from build123d import *

# Parameters (mm, degrees)
SKETCH_R        = 90
PAD_DEPTH       = 1.6
SKETCH001_R     = 90
SKETCH001_R_2   = 88
PAD001_DEPTH    = 20
SKETCH006_R     = 5.2
POCKET_DEPTH    = 6
PAD006_DEPTH    = 20
POCKET001_DEPTH = 8
SKETCH008_R     = 5.2
PAD007_DEPTH    = 1.8
SKETCH057_R     = 1.396673
SKETCH057_R_2   = 1.389292
SKETCH057_W     = 5
SKETCH057_H     = 5
PAD037_DEPTH    = 20


with BuildPart() as part:
    # Sketch → Pad (new body)
    with BuildSketch(Plane.XY):
        Circle(SKETCH_R)
    extrude(amount=PAD_DEPTH)

    # Sketch001 (on Face3 of Pad) → Pad001 (join)
    with BuildSketch(Plane.XY.offset(1.6)):
        Circle(SKETCH001_R)
        Circle(SKETCH001_R_2, mode=Mode.SUBTRACT)
    extrude(amount=PAD001_DEPTH)

    # Sketch006 (on Face2 of ShapeBinder) → Pocket (cut)
    with BuildSketch(Plane(origin=(0, 90, 8), x_dir=(1, 0, 0), z_dir=(0, 1, 0))):
        Circle(SKETCH006_R)
    extrude(amount=-POCKET_DEPTH, mode=Mode.SUBTRACT)

    # Sketch007 (on Face7 of Pocket) → Pad006 (join)
    with BuildSketch(Plane.XY.offset(1.6)):
        with BuildLine():
            ThreePointArc((7, 87.721149), (0, 88), (-7, 87.721149))
            Line((-7, 87.721149), (-7, 84))
            Line((-7, 84), (7, 84))
            Line((7, 84), (7, 87.721149))
        make_face()
    extrude(amount=PAD006_DEPTH)

    # Sketch006 (on Face2 of ShapeBinder) → Pocket001 (cut)
    with BuildSketch(Plane(origin=(0, 90, 8), x_dir=(1, 0, 0), z_dir=(0, 1, 0))):
        Circle(SKETCH006_R)
    extrude(amount=-POCKET001_DEPTH, mode=Mode.SUBTRACT)

    # Sketch008 (on Face13 of Pocket001) → Pad007 (join)
    with BuildSketch(Plane.XZ.offset(-84)):
        with Locations((0, 8)):
            Circle(SKETCH008_R)
        with BuildLine():
            ThreePointArc((1.843231, 4.45), (4, 8), (1.843231, 11.55))
            Line((-1.843231, 11.55), (1.843231, 11.55))
            ThreePointArc((-1.843231, 11.55), (-4, 8), (-1.843231, 4.45))
            Line((-1.843231, 4.45), (1.843231, 4.45))
        make_face(mode=Mode.SUBTRACT)
    extrude(amount=-PAD007_DEPTH)

    # Sketch057 (on Face10 of Pad007) → Pad037 (join)
    with BuildSketch(Plane.XY.offset(1.6)):
        with Locations((15.604022, 34.492405)):
            Circle(SKETCH057_R)
        with Locations((30.599703, -34.504681)):
            Circle(SKETCH057_R_2)
        with Locations((-34.349093, -62.155302)):
            Rectangle(SKETCH057_W, SKETCH057_H)
        with Locations((-9.349093, -62.155302)):
            Rectangle(SKETCH057_W, SKETCH057_H)
        with Locations((15.650907, -62.155302)):
            Rectangle(SKETCH057_W, SKETCH057_H)
        with Locations((40.650907, -62.155302)):
            Rectangle(SKETCH057_W, SKETCH057_H)
        with Locations((-59.349093, -37.155302)):
            Rectangle(SKETCH057_W, SKETCH057_H)
        with Locations((-34.349093, -37.155302)):
            Rectangle(SKETCH057_W, SKETCH057_H)
        with Locations((40.650907, -37.155302)):
            Rectangle(SKETCH057_W, SKETCH057_H)
        with Locations((65.650907, -37.155302)):
            Rectangle(SKETCH057_W, SKETCH057_H)
        with Locations((-59.349093, -12.155302)):
            Rectangle(SKETCH057_W, SKETCH057_H)
        with Locations((-34.349093, -12.155302)):
            Rectangle(SKETCH057_W, SKETCH057_H)
        with Locations((40.650907, -12.155302)):
            Rectangle(SKETCH057_W, SKETCH057_H)
        with Locations((65.650907, -12.155302)):
            Rectangle(SKETCH057_W, SKETCH057_H)
        with Locations((-59.349093, 12.844698)):
            Rectangle(SKETCH057_W, SKETCH057_H)
        with Locations((-34.349093, 12.844698)):
            Rectangle(SKETCH057_W, SKETCH057_H)
        with Locations((40.650907, 12.844698)):
            Rectangle(SKETCH057_W, SKETCH057_H)
        with Locations((65.650907, 12.844698)):
            Rectangle(SKETCH057_W, SKETCH057_H)
        with Locations((-59.349093, 37.844698)):
            Rectangle(SKETCH057_W, SKETCH057_H)
        with Locations((-34.349093, 37.844698)):
            Rectangle(SKETCH057_W, SKETCH057_H)
        with Locations((40.650907, 37.844698)):
            Rectangle(SKETCH057_W, SKETCH057_H)
        with Locations((65.650907, 37.844698)):
            Rectangle(SKETCH057_W, SKETCH057_H)
        with Locations((-34.349093, 62.844698)):
            Rectangle(SKETCH057_W, SKETCH057_H)
        with Locations((-9.349093, 62.844698)):
            Rectangle(SKETCH057_W, SKETCH057_H)
        with Locations((15.650907, 62.844698)):
            Rectangle(SKETCH057_W, SKETCH057_H)
        with Locations((40.650907, 62.844698)):
            Rectangle(SKETCH057_W, SKETCH057_H)
    extrude(amount=PAD037_DEPTH)


solid = part.part
Design review of the part built by this model. Coordinates are the model's own, in mm. A direction names the side the tool comes from. Give positions to 0.01 mm unless a question says otherwise; leave off trailing zeros. Order: outer loops, then holes, each group sorted by start corner. A loop starts at its lowest first (then second) coordinate and runs counter-clockwise, first axis right, second up.
1. Tool access review of faces 4 (the flat face through (-61.849, -12, 11)), 5 (the flat face through (0, 85.8, 4)): name each direction out of +Z, -Z, +X, -X, +Y, -Y from which nothing blocks a thin tool from reaching the whole face with its end or side.
Solution:
face 4: +Z
face 5: +Y
2. To check wall thickness, follow L1, parallel to X at y = -64.5, z = 18.5; L2, parallel to Y at x = 15, z = 20.75; L3, parallel to Z at x = 0, y = 89. State the ranges of each line that lie inside material, in increasing order.
Solution:
L1: x = -62.77 to -59.86, -36.85 to -31.85, -11.85 to -6.85, 13.15 to 18.15, 38.15 to 43.15, 59.86 to 62.77
L2: y = -88.74 to -86.71, -64.66 to -59.66, 33.23 to 35.75, 60.34 to 65.34, 86.71 to 88.74
L3: z = 0 to 2.8, 13.2 to 21.6
3. For pin 1 Ø4 at (x, z) = (-10.5, 16) entering from -Y; pin 2 Ø3 at (y, z) = (52, 10.5) entering from -X; pin 3 Ø4 at (y, z) = (-43, 3.5) entering from -X, all flat-tipped, find the tip position at first contact; note any pin that passes through.
Solution:
pin 1: stops at y = -89.6
pin 2: stops at x = -74.5
pin 3: stops at x = -80.12
4. Add section C-C, the plane y = 26. State the section outline as (x, z) points.
Solution:
outline: (-86.16, 0) - (86.16, 0) - (86.16, 21.6) - (84.07, 21.6) - (84.07, 1.6) - (-84.07, 1.6) - (-84.07, 21.6) - (-86.16, 21.6) - close
5. Add section A-A, the plane y = 0. State the section outline as (x, z) points, then the cut area to 3 significant figures.
Solution:
outline: (-90, 0) - (90, 0) - (90, 21.6) - (88, 21.6) - (88, 1.6) - (-88, 1.6) - (-88, 21.6) - (-90, 21.6) - close
area: 368 mm2
6. Add section B-B, the plane z = 19. State how many separate pieces and enclosed holes the cut face has, then the cut area to 3 significant figures.
Solution:
separate pieces: 27
enclosed holes: 1
area: 1,790 mm2
7. Mouldability with a two-part tool opening along X and no side actions: class faces 1 (the flat face through (38.151, -62, 11)), 2 (the flat face through (66, 35.345, 11)), 3 (the flat face through (-59, 38, 21.6)) as +X half, -X half, draft (parallel to the pull), parting line (faces both ways), or undercut.
Solution:
face 1: undercut
face 2: undercut
face 3: draft
